Source: three-view drawing plus pictorial views. Frame: mm from the lowest corner of the part. A direction names the side the tool comes from. Give positions to 0.01 mm unless a question says otherwise; leave off trailing zeros. Loops run counter-clockwise (first coordinate to the right, second up) from the corner with the lowest first, then second, coordinate; pieces in that order, holes last.
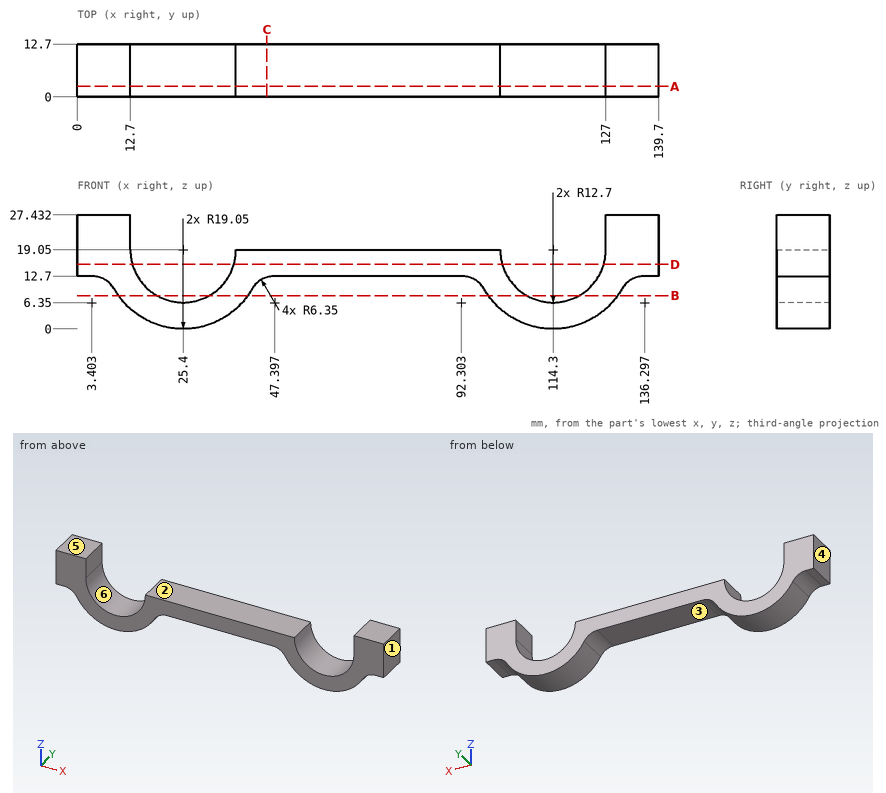
(1) Cut plane D-D (z = 15.5). Return the cut outline in (x, y).
Values follow:
outline: (0, 0) - (13.21, 0) - (13.21, 12.7) - (0, 12.7) - close; (37.59, 0) - (102.11, 0) - (102.11, 12.7) - (37.59, 12.7) - close; (126.49, 0) - (139.7, 0) - (139.7, 12.7) - (126.49, 12.7) - close
(2) Cut plane A-A (y = 2.5). Return the cut outline in (x, z) (3 decimals).
Values follow:
outline: (0, 12.7) - (3.403, 12.7) arc R6.35 cw to (8.902, 9.525) arc R19.05 ccw to (41.898, 9.525) arc R6.35 cw to (47.397, 12.7) - (92.303, 12.7) arc R6.35 cw to (97.802, 9.525) arc R19.05 ccw to (130.798, 9.525) arc R6.35 cw to (136.297, 12.7) - (139.7, 12.7) - (139.7, 27.432) - (127, 27.432) - (127, 19.05) arc R12.7 cw to (101.6, 19.05) - (38.1, 19.05) arc R12.7 cw to (12.7, 19.05) - (12.7, 27.432) - (0, 27.432) - close
(3) Reachability of the marked faces 1, 2 and 3 from +Z, -Z, +X, -X, +Y, -Y: full face, straight path, thin tool, end or side. Return the list, or none.
Values follow:
face 1: +Z, -Z, +X, +Y, -Y
face 2: +Z, +Y, -Y
face 3: -Z, +Y, -Y
(4) Ray query, probe 1 along X at (y, z) = (2, 22.5); probe 2 along X at (y, z) = (7, 15.25); probe 3 along X at (y, z) = (10, 16.25). Return the intervals inside material, ascending.
Values follow:
probe 1: x = 0 to 12.7, 127 to 139.7
probe 2: x = 0 to 13.28, 37.52 to 102.18, 126.42 to 139.7
probe 3: x = 0 to 13.01, 37.79 to 101.91, 126.69 to 139.7
(5) Mould query, pull axis X, two halves, no side actions, for the marked faces 4, 5 and 6. Classes: +X half, -X half, draft (parallel to the pull), parting line (faces both ways), or undercut.
Values follow:
face 4: -X half
face 5: draft
face 6: undercut
(6) Pin query (flat end, axial travel): pin 1 Ø10 at (x, z) = (117, 7) entering from -Y; pin 2 Ø3.5 at (x, y) = (138.5, 6) entering from -Z; pin 3 Ø6.5 at (x, y) = (58, 3.5) entering from +Z. Return the tip coordinate at first contact, or that it passes through.
Values follow:
pin 1: stops at y = 0
pin 2: stops at z = 12.7
pin 3: stops at z = 19.05
(7) Cut plane B-B (z = 8). Return the cut outline in (x, y).
Values follow:
outline: (9.88, 0) - (19.14, 0) - (19.14, 12.7) - (9.88, 12.7) - close; (31.66, 0) - (40.92, 0) - (40.92, 12.7) - (31.66, 12.7) - close; (98.78, 0) - (108.04, 0) - (108.04, 12.7) - (98.78, 12.7) - close; (120.56, 0) - (129.82, 0) - (129.82, 12.7) - (120.56, 12.7) - close
(8) Cut plane C-C (x = 45.5). Return the cut outline in (y, z), and give its area (3 significant figures).
Values follow:
outline: (0, 12.41) - (12.7, 12.41) - (12.7, 19.05) - (0, 19.05) - close
area: 84.3 mm2
